from build123d import *

# Parameters (mm, degrees)
BOSS_EXTRUDE1_DEPTH      = 13
BOSS_EXTRUDE1_DEPTH_BACK = 8
SKETCH2_W                = 56
SKETCH2_H                = 56
CUT_EXTRUDE1_DEPTH       = 12
CUT_EXTRUDE1_DEPTH_BACK  = 42.677331968
SKETCH1_R                = 18.5
SKETCH4_R                = 15
CUT_EXTRUDE2_DEPTH       = 42.677331968
CUT_EXTRUDE3_START       = -42.677331968
SKETCH5_W                = 12
SKETCH5_H                = 8
CUT_EXTRUDE3_DEPTH       = 54.677331968
SKETCH6_W                = 40.5
SKETCH6_H                = 40.5
CUT_EXTRUDE4_DEPTH       = 42.677331968
SKETCH3_R                = 1.05
CUT_EXTRUDE5_DEPTH       = 42.677331968
CIRPATTERN1_COUNT        = 4
SKETCH7_W                = 98
SKETCH7_H                = 21
BOSS_EXTRUDE2_DEPTH      = 2
BOSS_EXTRUDE3_DEPTH      = 16
SKETCH9_R                = 3.1
CUT_EXTRUDE6_DEPTH       = 69.183575735
SKETCH10_W               = 26
SKETCH10_H               = 9.75
CUT_EXTRUDE7_DEPTH       = 62.522353661
SKETCH11_R               = 1.6
CUT_EXTRUDE8_DEPTH       = 62.171888969
MIRROR4_COPY_1_SKETCH_R  = 1.6
MIRROR4_COPY_1_DEPTH     = 62.171888969
CIRPATTERN2_COUNT        = 4
CIRPATTERN3_COUNT        = 4


with BuildPart() as part:
    # Sketch2 → Boss-Extrude1 (new, two sides: drawn at the far end of the back side and taken through both)
    with BuildSketch(Plane.XY.offset(-BOSS_EXTRUDE1_DEPTH_BACK)):
        Rectangle(SKETCH2_W, SKETCH2_H)
    extrude(amount=BOSS_EXTRUDE1_DEPTH + BOSS_EXTRUDE1_DEPTH_BACK)

    # Sketch1 → Cut-Extrude1 (cut, two sides: drawn at the far end of the back side and taken through both)
    with BuildSketch(Plane.XY.offset(-CUT_EXTRUDE1_DEPTH_BACK)):
        Circle(SKETCH1_R)
    extrude(amount=CUT_EXTRUDE1_DEPTH + CUT_EXTRUDE1_DEPTH_BACK, mode=Mode.SUBTRACT)

    # Sketch4 → Cut-Extrude2 (cut, through all)
    with BuildSketch(Plane.XY):
        with Locations(Location((0, 0, 0), (0, 0, 180))):
            Circle(SKETCH4_R)
    extrude(amount=CUT_EXTRUDE2_DEPTH, mode=Mode.SUBTRACT)

    # Sketch5 → Cut-Extrude3 (cut)
    with BuildSketch(Plane.XY.offset(CUT_EXTRUDE3_START)):
        with Locations((0, 18)):
            Rectangle(SKETCH5_W, SKETCH5_H)
    cut_extrude3 = extrude(amount=CUT_EXTRUDE3_DEPTH, mode=Mode.SUBTRACT)

    # Sketch6 → Cut-Extrude4 (cut, through all)
    with BuildSketch(Plane.XY):
        Rectangle(SKETCH6_W, SKETCH6_H)
    extrude(amount=-CUT_EXTRUDE4_DEPTH, mode=Mode.SUBTRACT)

    # Sketch3 → Cut-Extrude5 (cut, symmetric)
    with BuildSketch(Plane.XY):
        with Locations((15, 15)):
            Circle(SKETCH3_R)
    cut_extrude5 = extrude(amount=CUT_EXTRUDE5_DEPTH, both=True, mode=Mode.SUBTRACT)

    # CirPattern1: Cut-Extrude5 ×4 about axis
    cirpattern1_axis = Axis((0, 0, 0), (0, 0, 1))
    for i in range(1, CIRPATTERN1_COUNT):
        add(cut_extrude5.rotate(cirpattern1_axis, i * 360 / CIRPATTERN1_COUNT), mode=Mode.SUBTRACT)

    # Sketch7 → Boss-Extrude2 (add)
    with BuildSketch(Plane.XZ.offset(28)):
        with Locations((0, 2.5)):
            Rectangle(SKETCH7_W, SKETCH7_H)
    extrude(amount=BOSS_EXTRUDE2_DEPTH)

    # Sketch8 → Boss-Extrude3 (add)
    with BuildSketch(Plane.XZ.offset(30)):
        Polygon((49, 13), (39, 13), (28, 13), (28, -8), (38, -8), (38, -22), (49, -22), align=None)
    boss_extrude3 = extrude(amount=-BOSS_EXTRUDE3_DEPTH)

    # Mirror1: Boss-Extrude3 across plane
    add(boss_extrude3.mirror(Plane(origin=(0, 0, 0), x_dir=(0, 0, 1), z_dir=(1, 0, 0))))

    # Sketch9 → Cut-Extrude6 (cut, through all)
    with BuildSketch(Plane(origin=(0, -14, 0), x_dir=(1, 0, 0), z_dir=(0, 1, 0))):
        with Locations(Location((-43.5, 16, 0), (0, 0, 270))):
            Circle(SKETCH9_R)
    cut_extrude6 = extrude(amount=-CUT_EXTRUDE6_DEPTH, mode=Mode.SUBTRACT)

    # Mirror2: Cut-Extrude6 across plane
    add(cut_extrude6.mirror(Plane(origin=(0, 0, 0), x_dir=(0, 0, 1), z_dir=(1, 0, 0))), mode=Mode.SUBTRACT)

    # Sketch10 → Cut-Extrude7 (cut, through all)
    with BuildSketch(Plane(origin=(0, 0, 0), x_dir=(-1, 0, 0), z_dir=(0, 0, -1))):
        with Locations((0, -25.125)):
            Rectangle(SKETCH10_W, SKETCH10_H)
    cut_extrude7 = extrude(amount=CUT_EXTRUDE7_DEPTH, mode=Mode.SUBTRACT)

    # Sketch11 → Cut-Extrude8 (cut, through all)
    with BuildSketch(Plane(origin=(0, 0, -8), x_dir=(-1, 0, 0), z_dir=(0, 0, -1))):
        with Locations((-23, 23)):
            Circle(SKETCH11_R)
    cut_extrude8 = extrude(amount=-CUT_EXTRUDE8_DEPTH, mode=Mode.SUBTRACT)

    # Mirror3: Cut-Extrude8 across plane
    add(cut_extrude8.mirror(Plane.ZX), mode=Mode.SUBTRACT)

    # Mirror4: Cut-Extrude8 across plane
    add(cut_extrude8.mirror(Plane(origin=(0, 0, 0), x_dir=(0, 0, 1), z_dir=(1, 0, 0))), mode=Mode.SUBTRACT)

    # Mirror4 copy 1 sketch → Mirror4 copy 1 (cut, through all)
    with BuildSketch(Plane(origin=(0, 0, -8), x_dir=(1, 0, 0), z_dir=(0, 0, -1))):
        with Locations((-23, 23)):
            Circle(MIRROR4_COPY_1_SKETCH_R)
    extrude(amount=-MIRROR4_COPY_1_DEPTH, mode=Mode.SUBTRACT)

    # CirPattern2: Cut-Extrude3 ×4 about axis
    cirpattern2_axis = Axis((0, 0, 0), (0, 0, 1))
    for i in range(1, CIRPATTERN2_COUNT):
        add(cut_extrude3.rotate(cirpattern2_axis, i * 360 / CIRPATTERN2_COUNT), mode=Mode.SUBTRACT)

    # CirPattern3: Cut-Extrude7 ×4 about axis
    cirpattern3_axis = Axis((0, 0, 0), (0, 0, 1))
    for i in range(1, CIRPATTERN3_COUNT):
        add(cut_extrude7.rotate(cirpattern3_axis, i * 360 / CIRPATTERN3_COUNT), mode=Mode.SUBTRACT)


solid = part.part
CAD build for the part. Positions are in the model's coordinates, mm. A direction names the side the tool comes from. Coordinates: 2 decimals unless noted, no trailing zeros. Write each loop counter-clockwise with the first axis right and the second up, starting at its lowest first coordinate (ties: lowest second). Pieces come first, ordered by that corner, then holes. Notation, with made-up numbers: M -16.75,-32.5 L 39.25,-32.5 A10 ccw 39.25,-14.5 Z; hole C 23,19 d3. An arc over 180 degrees is marked long. Return JSON: item names as keys, results as strings.
Item 1: Slice it at B-B, the plane x = -43.5. Write the cut outline in (y, z), and give its area (3 significant figures).
Findings below:
{"outline": "M -30,-22 L -14,-22 L -14,-19.1 L -30,-19.1 Z; M -30,-12.9 L -14,-12.9 L -14,13 L -30,13 Z", "area": "461 mm2"}
Item 2: Which spindle directions (+Z, -Z, +X, -X, +Y, -Y) get a long thin tool onto all of the face, cutting with end or side? Do faces 4 (the flat face through (13, 24, -4)), 5 (the flat face through (-22, 0, 6)), 6 (the flat face through (-28, 7, 5)), 7 (the cylindrical face through (-23.208, -24.586, 2.353)), 8 (the flat face through (28, 7, 5)). Say none if no direction does.
Findings below:
{"face 4": "-Z, +Y, -Y", "face 5": "-Z", "face 6": "+Z, -Z, -X, +Y", "face 7": "+Z, -Z", "face 8": "+Z, -Z, +X, +Y"}
Item 3: Drop flat-ended pins along their axis: pin 1 Ø12 at (x, y) = (25, 17) entering from -Z; pin 2 Ø13 at (y, z) = (-0.5, 6.5) entering from +X; pin 3 Ø13 at (y, z) = (3, 7.5) entering from -X. Give the stop position or say it passes through.
Findings below:
{"pin 1": "stops at z = -8", "pin 2": "stops at x = 28", "pin 3": "stops at x = -28"}
Item 4: Slice it at A-A, the plane z = -6. State how many separate pieces and enclosed holes the cut face has, and give its area (3 significant figures).
Findings below:
{"separate pieces": "4", "enclosed holes": "4", "area": "1,390 mm2"}
Item 5: Probe line 1 (Y direction, x = 23, z = 7); line 2 (X direction, y = -23, z = 5); line 3 (Y direction, x = -23, z = -3). List the from-to ranges inside material, lowest first. Write a range as from..to.
Findings below:
{"line 1": "y = -30..-24.6, -21.4..21.4, 24.6..28", "line 2": "x = -49..-24.6, -21.4..21.4, 24.6..49", "line 3": "y = -30..-24.6, -21.4..-13, 13..21.4, 24.6..28"}
Item 6: Two-plate mould, pull along Z, no slides. Class faces 1 (the flat face through (22, 0, 6)), 2 (the flat face through (3, 15, 12)), 3 (the cylindrical face through (40.426, -21.888, -16.404)): +Z half, -Z half, draft (parallel to the pull), parting line (faces both ways), or undercut.
Findings below:
{"face 1": "draft", "face 2": "-Z half", "face 3": "undercut"}
Item 7: Slice it at D-D, the plane z = -15. Write the cut outline in (x, y), and give its area (3 significant figures).
Findings below:
{"outline": "M -49,-30 L -46.43,-30 L -46.43,-14 L -49,-14 Z; M -40.57,-30 L -38,-30 L -38,-14 L -40.57,-14 Z; M 38,-30 L 40.57,-30 L 40.57,-14 L 38,-14 Z; M 46.43,-30 L 49,-30 L 49,-14 L 46.43,-14 Z", "area": "164 mm2"}
